Can you work these out from the model? Positions are in its coordinate system, mm. Round coordinates to 2 decimals unless told otherwise and drop trailing zeros. Order: outer loops, then holes, each group sorted by start corner. A loop starts at its lowest first (then second) coordinate and runs counter-clockwise, first axis right, second up.
Q1. If we section it at C-C (z = 3.25): Please give me the cut outline in (x, y), plus the area to 3 significant figures.
Q2. Will these pins go through, and if not, where does the flat tip stop? P1, Ø3, axis at y = -30.5, z = 12, coming from the +X side; P2, Ø1, axis at x = 98.5, z = 2, coming from the -Y side; P3, Ø2, axis at x = 16, z = 1.5, coming from the +Y side.
Q3. If I drill on line 1 (X direction, y = -29.5, z = 10.5); line 2 (Y direction, x = 44.5, z = 5.5); line 3 (Y direction, x = -13.5, z = 2.25), over which ranges is the centre line in solid material (lowest first)?
Q4. If we section it at B-B (z = 12): Please give me the cut outline in (x, y).
Q5. If we section it at A-A (x = -44): Please give me the cut outline in (y, z).
from build123d import *

# Parameters (mm, degrees)
F0_W     = 177.8
F0_H     = 101.6
F1_DEPTH = 14
F2_R     = 4
F3_R     = 6


with BuildPart() as f1:
    # F0 (on Top) → F1 (new body)
    with BuildSketch(Plane.XY):
        with Locations((30.6, -0.2)):
            Rectangle(F0_W, F0_H)
    extrude(amount=F1_DEPTH)

    # F2
    f2_edges = [f1.edges().sort_by_distance(p)[0] for p in [
        (-58.3, -0.2, 14),
        (30.6, 50.6, 14),
        (30.6, -51, 14),
        (119.5, -0.2, 14),
    ]]
    fillet(f2_edges, radius=F2_R)

    # F3
    f3_edges = [f1.edges().sort_by_distance(p)[0] for p in [
        (-58.3, -0.2, 0),
        (30.6, 50.6, 0),
        (30.6, -51, 0),
        (119.5, -0.2, 0),
    ]]
    fillet(f3_edges, radius=F3_R)


solid = f1.part
Solution:
1. outline: (-57.63, -50.33) - (118.83, -50.33) - (118.83, 49.93) - (-57.63, 49.93) - close
1. area: 17,700 mm2
2. P1: stops at x = 119.47
2. P2: stops at y = -49.87
2. P3: stops at y = 49.47
3. line 1: x = -58.27 to 119.47
3. line 2: y = -50.98 to 50.58
3. line 3: y = -49.68 to 49.28
4. outline: (-57.76, -50.46) - (118.96, -50.46) - (118.96, 50.06) - (-57.76, 50.06) - close
5. outline: (-51, 6) arc R6 ccw to (-45, 0) - (44.6, 0) arc R6 ccw to (50.6, 6) - (50.6, 10) arc R4 ccw to (46.6, 14) - (-47, 14) arc R4 ccw to (-51, 10) - close
